from build123d import *

# Parameters (mm, degrees)
CROQUIS1_R              = 1.75
SALIENTE_EXTRUIR1_DEPTH = 5
CROQUIS2_W              = 25
CROQUIS2_H              = 3
CROQUIS2_W_2            = 16.3
SALIENTE_EXTRUIR2_DEPTH = 21
CROQUIS4_W              = 3
CROQUIS4_H              = 5
SALIENTE_EXTRUIR3_DEPTH = 6
CROQUIS5_R              = 1.75
CORTAR_EXTRUIR2_DEPTH   = 90.541331239
CHAFL_N1_SIZE           = 6
CROQUIS6_W              = 25
CROQUIS6_H              = 3
SALIENTE_EXTRUIR4_DEPTH = 6
CROQUIS7_R              = 1.75
CROQUIS7_W              = 8
CROQUIS7_H              = 2
CORTAR_EXTRUIR3_DEPTH   = 69.693886191
CHAFL_N2_SIZE           = 3


with BuildPart() as part:
    # Croquis1 → Saliente-Extruir1 (new body)
    with BuildSketch(Plane(origin=(0, 0, 0), x_dir=(1, 0, 0), z_dir=(0, 1, 0))):
        Polygon((-36.3, 17.3), (36.3, 17.3), (41.3, 17.3), (41.3, 22.3), (-41.3, 22.3), (-41.3, -22.3), (41.3, -22.3), (41.3, -17.3), (36.3, -17.3), (-36.3, -17.3), align=None)
        with Locations(Location((-20, 20, 0), (0, 0, 270))):
            Circle(CROQUIS1_R, mode=Mode.SUBTRACT)
        with Locations(Location((20, 20, 0), (0, 0, 270))):
            Circle(CROQUIS1_R, mode=Mode.SUBTRACT)
        with Locations(Location((-20, -20, 0), (0, 0, 270))):
            Circle(CROQUIS1_R, mode=Mode.SUBTRACT)
        with Locations(Location((20, -20, 0), (0, 0, 270))):
            Circle(CROQUIS1_R, mode=Mode.SUBTRACT)
    extrude(amount=SALIENTE_EXTRUIR1_DEPTH)

    # Croquis2 → Saliente-Extruir2 (add)
    with BuildSketch(Plane(origin=(0, 5, 0), x_dir=(1, 0, 0), z_dir=(0, 1, 0))):
        Polygon((-39.3, 20.3), (-39.3, -20.3), (-25, -20.3), (-25, -17.3), (-36.3, -17.3), (-36.3, 17.3), (-25, 17.3), (-25, 20.3), align=None)
        with Locations((0, -20.8)):
            Rectangle(CROQUIS2_W, CROQUIS2_H)
        with Locations((0, 20.8)):
            Rectangle(CROQUIS2_W, CROQUIS2_H)
        with Locations((33.15, -20.8)):
            Rectangle(CROQUIS2_W_2, CROQUIS2_H)
        with Locations((33.15, 20.8)):
            Rectangle(CROQUIS2_W_2, CROQUIS2_H)
    extrude(amount=SALIENTE_EXTRUIR2_DEPTH)

    # Croquis4 → Saliente-Extruir3 (add)
    with BuildSketch(Plane(origin=(0, 26, 0), x_dir=(1, 0, 0), z_dir=(0, 1, 0))):
        with Locations((-37.8, 0)):
            Rectangle(CROQUIS4_W, CROQUIS4_H)
    extrude(amount=SALIENTE_EXTRUIR3_DEPTH)

    # Croquis5 → Cortar-Extruir2 (cut, through all)
    with BuildSketch(Plane.ZY.offset(39.3)):
        with Locations((0, 29)):
            Circle(CROQUIS5_R)
    extrude(amount=-CORTAR_EXTRUIR2_DEPTH, mode=Mode.SUBTRACT)

    # Chaflán1
    chafl_n1_edges = [part.edges().sort_by_distance(p)[0] for p in [
        (-37.8, 26, 2.5),
        (-37.8, 26, -2.5),
    ]]
    chamfer(chafl_n1_edges, length=CHAFL_N1_SIZE - 0.0001)  # a hair under: the kernel refuses the full size

    # Croquis6 → Saliente-Extruir4 (add)
    with BuildSketch(Plane(origin=(0, 26, 0), x_dir=(1, 0, 0), z_dir=(0, 1, 0))):
        with Locations((0, 20.8)):
            Rectangle(CROQUIS6_W, CROQUIS6_H)
        with Locations((0, -20.8)):
            Rectangle(CROQUIS6_W, CROQUIS6_H)
    extrude(amount=SALIENTE_EXTRUIR4_DEPTH)

    # Croquis7 → Cortar-Extruir3 (cut, through all)
    with BuildSketch(Plane(origin=(0, 0, -22.3), x_dir=(-1, 0, 0), z_dir=(0, 0, -1))):
        with Locations((0, 29)):
            Circle(CROQUIS7_R)
        with Locations((0, 21)):
            Rectangle(CROQUIS7_W, CROQUIS7_H)
        with Locations((0, 6)):
            Rectangle(CROQUIS7_W, CROQUIS7_H)
    extrude(amount=-CORTAR_EXTRUIR3_DEPTH, mode=Mode.SUBTRACT)

    # Chaflán2
    chafl_n2_edges = [part.edges().sort_by_distance(p)[0] for p in [
        (-12.5, 5, 20.8),
        (12.5, 5, 20.8),
        (-12.5, 5, -20.8),
        (12.5, 5, -20.8),
    ]]
    chamfer(chafl_n2_edges, length=CHAFL_N2_SIZE)


solid = part.part
Geometry: final body of the model. Coordinates: model frame, mm. A direction names the side the tool comes from. Give positions to 0.01 mm unless a question says otherwise; leave off trailing zeros. Write each loop counter-clockwise with the first axis right and the second up, starting at its lowest first coordinate (ties: lowest second). Pieces come first, ordered by that corner, then holes.
(1) Cut plane D-D, the plane x = -35.5. Return loops of the section in (y, z).
(2) Access query for faces 4 (the flat face through (-32, 15, 20.3)), 5 (the flat face through (-12.5, 20, -21)), 6 (the cylindrical face through (21.735, 2.465, -20.228)), 7 (the flat face through (0, 22, -21)), 8 (the flat face through (33, 15, 19.3)). Directions: +Z, -Z, +X, -X, +Y, -Y. A direction counts if a zero-diameter tool reaches every point of the face in a straight line with its end or side. Return the directions, or none.
(3) Ray query, line 1 (X direction, y = 3.6, z = -20); line 2 (Z direction, x = 11, y = 10.5); line 3 (Z direction, x = 21, y = 2.5). Return the intervals inside material, ascending.
(4) Mould query, pull axis Z, two halves, no side actions, for faces 1 (the flat face through (-36.3, 12, 0)), 2 (the flat face through (-4, 6, -21)), 3 (the flat face through (-32, 15, -20.3)). Classes: released by +Z, released by -Z, zero draft, split by the parting line, or undercut.
(5) Cut plane B-B, the plane z = 0. Return loops of the section in (x, y).
(6) Cut plane C-C, the plane x = 0. Give the number of separate pieces and of enclosed holes in the cut face, then the cut area to 3 significant figures.
(7) First-contact query: P1, Ø2.5, axis at x = 30.5, z = 21, coming from the +Y side; P2, Ø2, axis at x = 13.5, z = -16.5, coming from the +Y side; P3, Ø6, axis at y = 19, z = -15, coming from the +X side. Flat tips, straight axial feed; report the tip coordinate or a pass-through.
(8) Cut plane A-A, the plane y = 13. Return loops of the section in (x, z).
Values follow:
1. outline: (0, -22.3) - (5, -22.3) - (5, -20.3) - (26, -20.3) - (26, -17.3) - (0, -17.3) - close; (0, 17.3) - (26, 17.3) - (26, 20.3) - (5, 20.3) - (5, 22.3) - (0, 22.3) - close
2. face 4: +Z, -X, +Y
2. face 5: +Z, -Z, +Y
2. face 6: +Y, -Y
2. face 7: +Z, -Z
2. face 8: +X, +Y
3. line 1: x = -41.3 to -21.75, -18.25 to 18.25, 21.75 to 41.3
3. line 2: z = -22.3 to -19.3, 19.3 to 22.3
3. line 3: z = -22.3 to -21.44, -18.56 to -17.3, 17.3 to 18.56, 21.44 to 22.3
4. face 1: undercut
4. face 2: zero draft
4. face 3: released by -Z
5. outline: (-41.3, 0) - (-36.3, 0) - (-36.3, 27.25) - (-39.3, 27.25) - (-39.3, 5) - (-41.3, 5) - close; (-39.3, 30.75) - (-36.3, 30.75) - (-36.3, 32) - (-39.3, 32) - close
6. separate pieces: 8
6. enclosed holes: 0
6. area: 167 mm2
7. P1: stops at y = 26
7. P2: stops at y = 5
7. P3: stops at x = -25
8. outline: (-39.3, -20.3) - (-25, -20.3) - (-25, -17.3) - (-36.3, -17.3) - (-36.3, 17.3) - (-25, 17.3) - (-25, 20.3) - (-39.3, 20.3) - close; (-12.5, -22.3) - (12.5, -22.3) - (12.5, -19.3) - (-12.5, -19.3) - close; (-12.5, 19.3) - (12.5, 19.3) - (12.5, 22.3) - (-12.5, 22.3) - close; (25, -22.3) - (41.3, -22.3) - (41.3, -19.3) - (25, -19.3) - close; (25, 19.3) - (41.3, 19.3) - (41.3, 22.3) - (25, 22.3) - close
